```python
from build123d import *

# Parameters (mm, degrees)
SKETCH1_R           = 65.235026919
SKETCH1_R_2         = 4.95
BOSS_EXTRUDE4_DEPTH = 10
SKETCH1_5_R         = 4.95
SKETCH1_5_R_2       = 5
BOSS_EXTRUDE5_DEPTH = 20


with BuildPart() as part:
    # Sketch1 → Boss-Extrude4 (new body)
    with BuildSketch(Plane(origin=(0, 0, 0), x_dir=(1, 0, 0), z_dir=(0, 1, 0))):
        with Locations(Location((0, 0, 0), (0, 0, 270))):  # turned: the seam where the file's is
            Circle(SKETCH1_R)
        with Locations(Location((0, 57.735026919, 0), (0, 0, 270))):  # turned: the seam where the file's is
            Circle(SKETCH1_R_2, mode=Mode.SUBTRACT)
        with BuildLine():
            ThreePointArc((-40.989114073, 28.69280839), (0, -50.033835809), (40.989114073, 28.69280839))
            ThreePointArc((40.989114073, 28.69280839), (0, 7.5), (-40.989114073, 28.69280839))
        make_face(mode=Mode.SUBTRACT)
    extrude(amount=BOSS_EXTRUDE4_DEPTH)

    # Sketch1_5 → Boss-Extrude5 (add)
    with BuildSketch(Plane(origin=(0, 0, 0), x_dir=(1, 0, 0), z_dir=(0, 1, 0))):
        with Locations(Location((0, 57.735026919, 0), (0, 0, 270))):  # turned: the seam where the file's is
            Circle(SKETCH1_5_R)
        with BuildLine():
            ThreePointArc((-40.989114073, 28.69280839), (0, -50.033835809), (40.989114073, 28.69280839))
            ThreePointArc((40.989114073, 28.69280839), (0, 7.5), (-40.989114073, 28.69280839))
        make_face()
        with Locations(Location((0, 0, 0), (0, 0, 270))):  # turned: the seam where the file's is
            Circle(SKETCH1_5_R_2, mode=Mode.SUBTRACT)
    extrude(amount=BOSS_EXTRUDE5_DEPTH)


solid = part.part
```
Model file for the job. Use its own axes, mm. A direction names the side the tool comes from. Give positions to 0.01 mm unless a question says otherwise; leave off trailing zeros. Loops run counter-clockwise (first coordinate to the right, second up) from the corner with the lowest first, then second, coordinate; pieces in that order, holes last. Notation, with made-up numbers: (3, 66.5) - (18, 66.5) arc R21 cw to (18, 72.5) - close; hole circle Ø10 at (53, 59.25). An arc over 180 degrees is marked (long way). One line per item, written item: value. Start each with the question number.
1. Pull direction X, two halves, no side cores. Call faces 3 (the cylindrical face through (-1.53, 14.93, 50.01)), 4 (the cylindrical face through (-4.88, 9.86, -1.08)), 5 (the flat face through (-1, 20, 10)): pulls with the +X half, pulls with the -X half, needs draft (parallel to the pull), parting line crosses it, or undercut.
2. Pin check, flat tips, straight feed: pin 1 (12 mm diameter, centred on x = -17.5, y = 2.5, fed in from +Z); pin 2 (3 mm diameter, centred on x = 23.5, y = 5, fed in from -Z); pin 3 (2 mm diameter, centred on y = 10.5, z = 50, fed in from -X); pin 4 (6 mm diameter, centred on x = 0, z = 0, fed in from -Y). Stop position of each tip, or through.
3. Probe L1, parallel to X at y = 8, z = 0; L2, parallel to X at y = 19, z = -58; L3, parallel to X at y = 10.75, z = 0. List the from-to ranges inside material, lowest first. Write a range as from..to.
4. Slice it at C-C (y = 11.5). List the corners of the cut face in (x, z), plus the area to 3 significant figures.
5. Slice it at A-A (z = 0). List the corners of the cut face in (x, y), plus the area to 3 significant figures.
6. Slice it at D-D (y = 3.5). List the corners of the cut face in (x, z), plus the area to 3 significant figures.
7. Which spindle directions (+Z, -Z, +X, -X, +Y, -Y) get a long thin tool onto all of the face, cutting with end or side? Do faces 1 (the flat face through (0, 20, -58)), 2 (the flat face through (1, 10, -15)). Say none if no direction does.
8. Slice it at B-B (x = 0). List the corners of the cut face in (y, z).
Solution:
1. face 3: parting line crosses it
1. face 4: undercut
1. face 5: needs draft
2. pin 1: stops at z = 64.21
2. pin 2: stops at z = -61.41
2. pin 3: stops at x = -42.91
2. pin 4: passes through
3. L1: x = -65.24..-5, 5..65.24
3. L2: x = -4.94..4.94
3. L3: x = -50.03..-5, 5..50.03
4. outline: (-40.99, -28.69) arc R50.24 cw to (40.99, -28.69) arc R50.03 ccw (long way) to start; circle Ø9.9 at (0, -57.74); hole circle Ø10 at (0, 0)
4. area: 5,420 mm^2
5. outline: (-65.24, 0) - (-5, 0) - (-5, 20) - (-50.03, 20) - (-50.03, 10) - (-65.24, 10) - close; (5, 0) - (65.24, 0) - (65.24, 10) - (50.03, 10) - (50.03, 20) - (5, 20) - close
5. area: 2,110 mm^2
6. outline: circle Ø130.47 at (0, 0); hole circle Ø10 at (0, 0)
6. area: 13,300 mm^2
7. face 1: +Z, -Z, +X, -X, +Y
7. face 2: +Y
8. outline: (0, -65.24) - (10, -65.24) - (10, -62.69) - (20, -62.69) - (20, -52.79) - (10, -52.79) - (10, -7.5) - (20, -7.5) - (20, -5) - (0, -5) - close; (0, 5) - (20, 5) - (20, 50.03) - (10, 50.03) - (10, 65.24) - (0, 65.24) - close
